Autodesk Inventor part; units mm, degrees
ref_plane "YZ Plane" through (0, 0, 0) normal (1, 0, 0) x (0, 1, 0)
ref_plane "XZ Plane" through (0, 0, 0) normal (0, 1, 0) x (-1, 0, 0)
ref_plane "XY Plane" through (0, 0, 0) normal (0, 0, 1) x (1, 0, 0)
sketch "Sketch20" plane through (0, 0, 0) normal (0, 1, 0) x (-1, 0, 0)
  line L0 (0, 0) -> (40, 0)
  line L1 (40, 0) -> (40, -45)
  line L2 (40, -45) -> (0, -45)
  line L3 (0, -45) -> (0, 0)
  line L4 (40, -45) -> (30, -45)
  line L5 (30, -45) -> (30, -35)
  line L6 (0, -45) -> (10, -45)
  line L7 (10, -45) -> (10, -35)
  circle A0 centre (30, -35) radius 3
  circle A1 centre (10, -35) radius 3
  dimension "d117" = 40
  dimension "d118" = 45
  dimension "d119" = 10
  dimension "d120" = 10
  dimension "d121" = 10
  dimension "d122" = 10
  dimension "d123" = 6
  dimension "d124" = 6
extrude "Extrusion20" add sketch "Sketch20" along normal blind 3
fillet "Fillet6" radius 5 4 edges at (0, 1.5, 0) (-40, 1.5, 0) (0, 1.5, -45) (-40, 1.5, -45)
properties part number "MagnetHolder_Special"
Build history of the part. All positions in model axes, mm. Round coordinates to 2 decimals unless told otherwise and drop trailing zeros. Order: outer loops, then holes, each group sorted by start corner. A loop starts at its lowest first (then second) coordinate and runs counter-clockwise, first axis right, second up. Notation, with made-up numbers: M 63,18.5 L 111,18.5 A19 cw 111,27.5 Z; hole C 37.25,7 d10. An arc over 180 degrees is marked long. Use CSV: the item, a comma, the result in double quotes. Start each with the question number.
(1) Cut at C-C on y = 1.6. List the corners of the cut face in (x, z).
(2) Cut at D-D on x = -27.5. List the corners of the cut face in (y, z), then the cut area to 3 significant figures.
(3) Drill centre lines: probe 1 along X at (y, z) = (1.3, -35); probe 2 along Z at (x, y) = (-30, 1.8); probe 3 along X at (y, z) = (2.85, -33). Where is each one in solid material? Low to high.
(4) Cut at B-B on z = -35. List the corners of the cut face in (x, y), then the cut area to 3 significant figures.
(5) Cut at A-A on x = -10. List the corners of the cut face in (y, z), then the cut area to 3 significant figures.
(6) Mould opens along Z. For faces 1 (the face through (-20, 0, -22)), 2 (the face through (-27.79, 1.48, -37.03)), 3 (the face through (-38, 2, -44)), 4 (the face through (-10, 1, -38)) say: +Z half, -Z half, draft (parallel to the pull), parting line (faces both ways), or undercut.
Findings:
1,outline,"M -40,-40 A5 ccw -35,-45 L -5,-45 A5 ccw 0,-40 L 0,-5 A5 ccw -5,0 L -35,0 A5 ccw -40,-5 Z; hole C -30,-35 d6; hole C -10,-35 d6"
2,outline,"M 0,-45 L 3,-45 L 3,-36.66 L 0,-36.66 Z; M 0,-33.34 L 3,-33.34 L 3,0 L 0,0 Z"
2,area,"125 mm^2"
3,probe 1,"x = -40 to -33, -27 to -13, -7 to 0"
3,probe 2,"z = -45 to -38, -32 to 0"
3,probe 3,"x = -40 to -32.24, -27.76 to -12.24, -7.76 to 0"
4,outline,"M -40,0 L -33,0 L -33,3 L -40,3 Z; M -27,0 L -13,0 L -13,3 L -27,3 Z; M -7,0 L 0,0 L 0,3 L -7,3 Z"
4,area,"84.0 mm^2"
5,outline,"M 0,-45 L 3,-45 L 3,-38 L 0,-38 Z; M 0,-32 L 3,-32 L 3,0 L 0,0 Z"
5,area,"117 mm^2"
6,face 1,"draft"
6,face 2,"undercut"
6,face 3,"-Z half"
6,face 4,"undercut"
